Drawing for the job (mm, zero at the part's lowest x, y, z). A direction names the side the tool comes from. Coordinates: 2 decimals unless noted, no trailing zeros. Order: outer loops, then holes, each group sorted by start corner. A loop starts at its lowest first (then second) coordinate and runs counter-clockwise, first axis right, second up.
1) Cut at C-C (z = 20.5). List the corners of the cut face in (x, y).
2) Tool access for the marked faces 1 and 2: list every direction of +Z, -Z, +X, -X, +Y, -Y with a clear straight run to the whole face (end or side of a thin tool).
3) Wall check: L1, parallel to X at y = 3, z = 11; L2, parallel to Y at x = 0.85, z = 36.5; L3, parallel to Y at x = 19.65, z = 21. Give the ranges that are in metal, low to high.
4) Mould opens along X. For the marked faces 3, 4 and 5 say: +X half, -X half, draft (parallel to the pull), parting line (faces both ways), or undercut.
5) Cut at B-B (y = 2.25). List the corners of the cut face in (x, z), and give its area (3 significant figures).
6) Pin check, flat tips, straight feed: pin 1 Ø4 at (x, z) = (11.5, 34) entering from -Y; pin 2 Ø5 at (x, z) = (8.5, 21.5) entering from +Y. Stop position of each tip, or through.
7) Cut at A-A (z = 5.5). List the corners of the cut face in (x, y).
8) Cut at D-D (y = 4.5). List the corners of the cut face in (x, z).
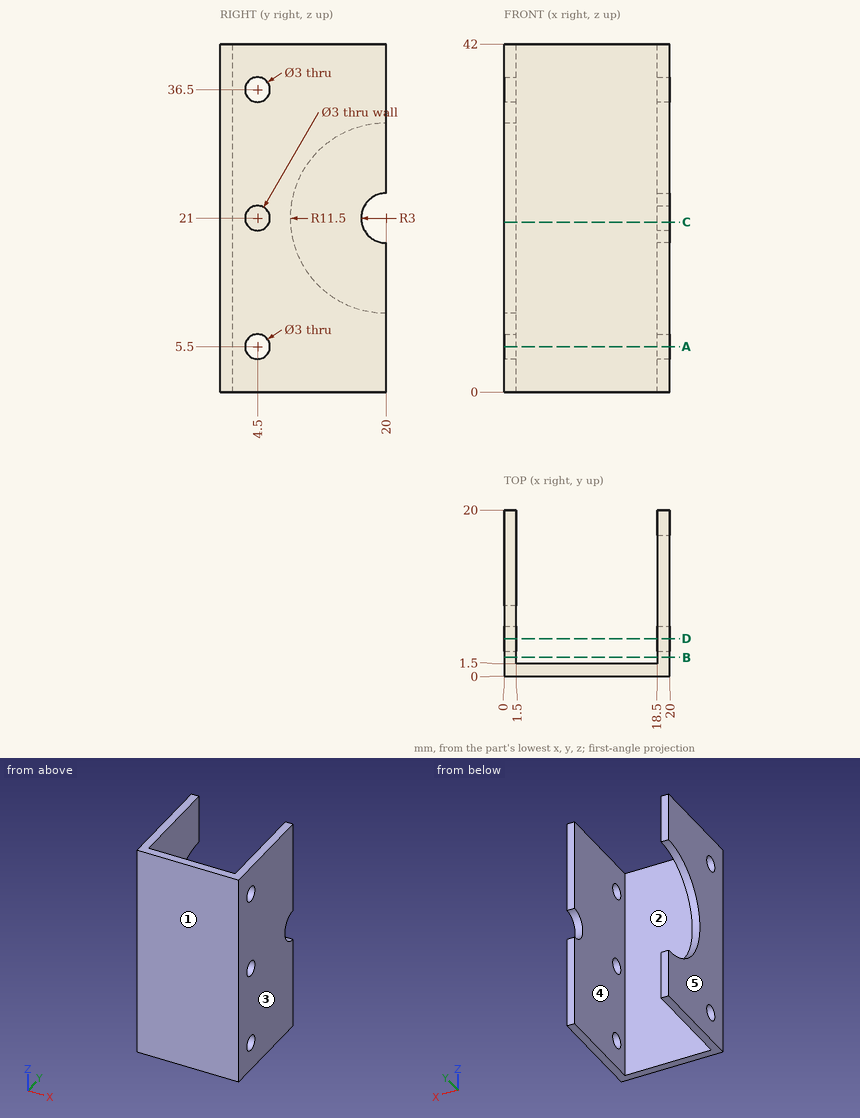
Geometry check:
1. outline: (0, 0) - (20, 0) - (20, 3.09) - (18.5, 3.09) - (18.5, 1.5) - (1.5, 1.5) - (1.5, 8.51) - (0, 8.51) - close; (18.5, 5.91) - (20, 5.91) - (20, 17.04) - (18.5, 17.04) - close
2. face 1: +Z, -Z, +X, -X, -Y
2. face 2: +Z, -Z, +Y
3. L1: x = 0 to 1.5, 18.5 to 20
3. L2: y = 0 to 3, 6 to 20
3. L3: y = 0 to 3, 6 to 17
4. face 3: +X half
4. face 4: undercut
4. face 5: -X half
5. outline: (0, 0) - (1.5, 0) - (1.5, 42) - (0, 42) - close; (18.5, 0) - (20, 0) - (20, 42) - (18.5, 42) - close
5. area: 126 mm2
6. pin 1: stops at y = 0
6. pin 2: stops at y = 1.5
7. outline: (0, 0) - (20, 0) - (20, 3) - (18.5, 3) - (18.5, 1.5) - (1.5, 1.5) - (1.5, 3) - (0, 3) - close; (0, 6) - (1.5, 6) - (1.5, 20) - (0, 20) - close; (18.5, 6) - (20, 6) - (20, 20) - (18.5, 20) - close
8. outline: (0, 0) - (1.5, 0) - (1.5, 4) - (0, 4) - close; (0, 7) - (1.5, 7) - (1.5, 35) - (0, 35) - close; (0, 38) - (1.5, 38) - (1.5, 42) - (0, 42) - close; (18.5, 0) - (20, 0) - (20, 4) - (18.5, 4) - close; (18.5, 7) - (20, 7) - (20, 19.5) - (18.5, 19.5) - close; (18.5, 22.5) - (20, 22.5) - (20, 35) - (18.5, 35) - close; (18.5, 38) - (20, 38) - (20, 42) - (18.5, 42) - close
